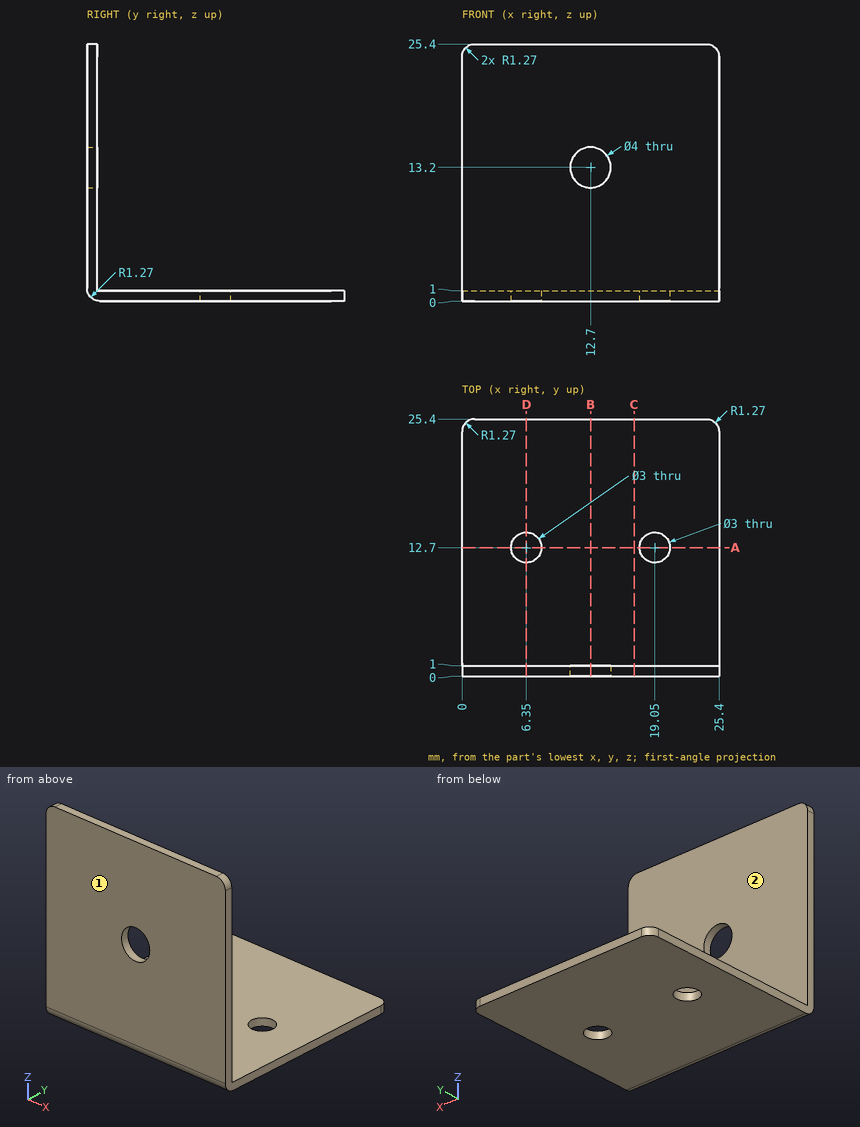
The figure shows three views and two pictorial views of one solid part (mm, origin at its lowest corner). Answer the questions. A direction names the side the tool comes from. Give positions to 0.01 mm unless a question says otherwise; leave off trailing zeros. Loops run counter-clockwise (first coordinate to the right, second up) from the corner with the lowest first, then second, coordinate; pieces in that order, holes last. Notation, with made-up numbers: (5.25, 69) -> (10.25, 69) arc R19 cw to (10.25, 92) -> close; hole circle Ø8 at (-6.5, 60). An arc over 180 degrees is marked (long way). Put each result on its own line as item: value. Start each with the question number.
Item 1: Which of the six approach directions +Z, -Z, +X, -X, +Y, -Y give full straight-line access (tool end or side, diameter ignored) to the marked faces 1 and 2?
Item 2: The part is cut by section D-D (x = 6.35). Give the vertices of the cut face in (y, z).
Item 3: The part is cut by section A-A (y = 12.7). Give the vertices of the cut face in (x, z).
Item 4: The part is cut by section C-C (x = 17). Give the vertices of the cut face in (y, z).
Item 5: Each of these flat-tipped pins is pushed along its axis until it touches: P1, Ø7.5, axis at x = 16.5, y = 18, coming from the +Z side; P2, Ø5, axis at x = 22.5, z = 13.5, coming from the +Y side. Where does it stop, or does it pass through?
Item 6: The part is cut by section B-B (x = 12.7). Give the vertices of the cut face in (y, z), then the cut area to 3 significant figures.
Item 7: Find the intervals of material crossed by L1, parallel to X at y = 12.7, z = 0.4; L2, parallel to Z at x = 16.5, y = 12.75, in increasing order. Write a range as [from, to].
Answers below:
1. face 1: +Z, -Z, +X, -X, -Y
1. face 2: +Z, +X, -X, +Y
2. outline: (0, 1.27) arc R1.27 ccw to (1.27, 0) -> (11.2, 0) -> (11.2, 1) -> (1, 1) -> (1, 25.4) -> (0, 25.4) -> close; (14.2, 0) -> (25.4, 0) -> (25.4, 1) -> (14.2, 1) -> close
3. outline: (0, 0) -> (4.85, 0) -> (4.85, 1) -> (0, 1) -> close; (7.85, 0) -> (17.55, 0) -> (17.55, 1) -> (7.85, 1) -> close; (20.55, 0) -> (25.4, 0) -> (25.4, 1) -> (20.55, 1) -> close
4. outline: (0, 1.27) arc R1.27 ccw to (1.27, 0) -> (25.4, 0) -> (25.4, 1) -> (1, 1) -> (1, 25.4) -> (0, 25.4) -> close
5. P1: z = 1
5. P2: y = 1
6. outline: (0, 1.27) arc R1.27 ccw to (1.27, 0) -> (25.4, 0) -> (25.4, 1) -> (1, 1) -> (1, 11.2) -> (0, 11.2) -> close; (0, 15.2) -> (1, 15.2) -> (1, 25.4) -> (0, 25.4) -> close
6. area: 45.5 mm2
7. L1: [0, 4.85], [7.85, 17.55], [20.55, 25.4]
7. L2: [0, 1]
